```python
from build123d import *

# Parameters (mm, degrees)
SKETCH1_R           = 18.5
BOSS_EXTRUDE1_DEPTH = 5
SKETCH2_R           = 22
SKETCH2_R_2         = 18.5
BOSS_EXTRUDE2_DEPTH = 21
CHAMFER1_SIZE       = 1.5


with BuildPart() as part:
    # Sketch1 → Boss-Extrude1 (new, symmetric)
    with BuildSketch(Plane(origin=(0, 0, 0), x_dir=(1, 0, 0), z_dir=(0, 1, 0))):
        Polygon((15.011106999, -26), (30.022213998, 0), (15.011106999, 26), (-15.011106999, 26), (-30.022213998, 0), (-15.011106999, -26), align=None)
        with Locations(Location((0, 0, 0), (0, 0, 270))):
            Circle(SKETCH1_R, mode=Mode.SUBTRACT)
    extrude(amount=BOSS_EXTRUDE1_DEPTH, both=True)

    # Sketch2 → Boss-Extrude2 (add, symmetric)
    with BuildSketch(Plane(origin=(0, 0, 0), x_dir=(1, 0, 0), z_dir=(0, 1, 0))):
        with Locations(Location((0, 0, 0), (0, 0, 90))):
            Circle(SKETCH2_R)
        with Locations(Location((0, 0, 0), (0, 0, 270))):
            Circle(SKETCH2_R_2, mode=Mode.SUBTRACT)
    extrude(amount=BOSS_EXTRUDE2_DEPTH, both=True)

    # Chamfer1
    chamfer1_edges = [part.edges().sort_by_distance(p)[0] for p in [
        (0, -21, 22),
        (0, 21, 22),
    ]]
    chamfer(chamfer1_edges, length=CHAMFER1_SIZE)


solid = part.part
```
For this review, take the finished solid that the model builds, in its own axes (mm). A direction names the side the tool comes from. Round coordinates to 2 decimals unless told otherwise and drop trailing zeros. Write each loop counter-clockwise with the first axis right and the second up, starting at its lowest first coordinate (ties: lowest second). Pieces come first, ordered by that corner, then holes. Notation, with made-up numbers: M 57,-30.75 L 65,-30.75 A31 cw 65,5.25 Z; hole C -0.75,64 d10. An arc over 180 degrees is marked long. One line per item, written item: value. Start each with the question number.
(1) We need section B-B (y = 2.5). Give the boundary of the cut face in (x, z), and give its area (3 significant figures).
(2) The part is to be moulded in two halves that separate along X. For faces 1 (the flat face through (20, 5, -10)), 2 (the cylindrical face through (-7.086, -0.294, 17.089)), 3 (the flat face through (22.4, 0.1, 13.2)), say which applies: released by +X, released by -X, zero draft, split by the parting line, or undercut.
(3) We need section C-C (y = -11). Give the boundary of the cut face in (x, z).
(4) Wall thickness on line 1 (X direction, y = -1, z = 0); line 2 (X direction, y = 11, z = 0); line 3 (Y direction, x = 19.5, z = -12): over which ranges is each line inside the solid? List them lowest first.
(5) We need section A-A (x = 0). Give the boundary of the cut face in (y, z).
(6) Machinability: for faces 4 (the flat face through (20, -5, -10)), 5 (the cylindrical face through (21.477, 12.352, 4.769)), 6 (the flat face through (-22.4, 0.1, -13.2)), which of the approach directions +Z, -Z, +X, -X, +Y, -Y give a long, thin tool a straight path to every point of the face, cutting with its end or side? Answer none if there is none.
(7) Insertion check: pin 1 (2 mm diameter, centred on x = 2.5, y = -12.5, fed in from -Z); pin 2 (3 mm diameter, centred on x = 18.5, y = -16.5, fed in from -Z); pin 3 (10 mm diameter, centred on x = -6.5, y = -15, fed in from +Z). Each pin has a flat end and moves straight along its axis. Give the tip position at first contact, or say it passes through.
Result:
1. outline: M -30.02,0 L -15.01,-26 L 15.01,-26 L 30.02,0 L 15.01,26 L -15.01,26 Z; hole C 0,0 d37
1. area: 1,270 mm²
2. face 1: zero draft
2. face 2: undercut
2. face 3: released by +X
3. outline: C 0,0 d44; hole C 0,0 d37
4. line 1: -30.02 to -18.5, 18.5 to 30.02
4. line 2: -22 to -18.5, 18.5 to 22
4. line 3: -5 to 5
5. outline: M -21,-20.5 L -19.5,-22 L -5,-22 L -5,-26 L 5,-26 L 5,-22 L 19.5,-22 L 21,-20.5 L 21,-18.5 L -21,-18.5 Z; M -21,18.5 L 21,18.5 L 21,20.5 L 19.5,22 L 5,22 L 5,26 L -5,26 L -5,22 L -19.5,22 L -21,20.5 Z
6. face 4: -Y
6. face 5: +Y
6. face 6: -Z, -X, +Y, -Y
7. pin 1: z = -21.95
7. pin 2: z = -13.96
7. pin 3: z = 21.95
